Could you check a few things on this model? Use its own coordinates, in mm. A direction names the side the tool comes from. Coordinates: 2 decimals unless noted, no trailing zeros. Loops run counter-clockwise (first coordinate to the right, second up) from the corner with the lowest first, then second, coordinate; pieces in that order, holes last. Notation, with made-up numbers: (23.5, 75) - (44.5, 75) arc R23 cw to (44.5, 103) - close; hole circle Ø9 at (3, 29). An arc over 180 degrees is marked (long way). Use CSV: the item, a comma, the result in double quotes.
from build123d import *

# Parameters (mm, degrees)
SKETCH1_W               = 139
SKETCH1_H               = 160
BOSS_EXTRUDE1_DEPTH     = 5
SKETCH2_W               = 16
SKETCH2_H               = 16
CUT_EXTRUDE1_DEPTH      = 107.090763029
SKETCH3_R               = 2.2
CUT_EXTRUDE2_DEPTH      = 107.090763029
SKETCH4_R               = 2.2
CUT_EXTRUDE3_DEPTH      = 107.090763029
LPATTERN1_COUNT         = 4
LPATTERN1_PITCH         = 35
MIRROR2_COPY_1_SKETCH_R = 2.2
MIRROR2_COPY_1_DEPTH    = 107.090763029
MIRROR2_COPY_2_SKETCH_R = 2.2
MIRROR2_COPY_2_DEPTH    = 107.090763029
MIRROR2_COPY_3_SKETCH_R = 2.2
MIRROR2_COPY_3_DEPTH    = 107.090763029
SKETCH5_R               = 2.2
CUT_EXTRUDE4_DEPTH      = 107.090763029
SKETCH10_W              = 109
SKETCH10_H              = 15
BOSS_EXTRUDE2_DEPTH     = 5
SKETCH9_W               = 55
SKETCH9_H               = 104
CUT_EXTRUDE5_DEPTH      = 118.814472795
SKETCH11_W              = 55
SKETCH11_H              = 5
BOSS_EXTRUDE3_DEPTH     = 60
SKETCH12_R              = 1.375
CUT_EXTRUDE6_DEPTH      = 153.368796018
CUT_EXTRUDE7_REACH      = 154.369
SKETCH13_R              = 1.375
CUT_EXTRUDE8_REACH      = 196.821
SKETCH14_R              = 1.375
FILLET1_R               = 10
FILLET2_R               = 10


with BuildPart() as part:
    # Sketch1 → Boss-Extrude1 (new body)
    with BuildSketch(Plane(origin=(0, 0, 0), x_dir=(1, 0, 0), z_dir=(0, 1, 0))):
        Rectangle(SKETCH1_W, SKETCH1_H)
    extrude(amount=BOSS_EXTRUDE1_DEPTH)

    # Sketch2 → Cut-Extrude1 (cut, through all)
    with BuildSketch(Plane(origin=(0, 5, 0), x_dir=(1, 0, 0), z_dir=(0, 1, 0))):
        with Locations((-61.5, -72)):
            Rectangle(SKETCH2_W, SKETCH2_H)
    cut_extrude1 = extrude(amount=-CUT_EXTRUDE1_DEPTH, mode=Mode.SUBTRACT)

    # Mirror1: Cut-Extrude1 across plane
    add(cut_extrude1.mirror(Plane(origin=(0, 0, 0), x_dir=(0, 0, 1), z_dir=(1, 0, 0))), mode=Mode.SUBTRACT)

    # Sketch3 → Cut-Extrude2 (cut, through all)
    with BuildSketch(Plane(origin=(0, 5, 0), x_dir=(1, 0, 0), z_dir=(0, 1, 0))):
        with Locations(Location((0, -72.5, 0), (0, 0, 270))):
            Circle(SKETCH3_R)
        with Locations(Location((-25, -72.5, 0), (0, 0, 270))):
            Circle(SKETCH3_R)
        with Locations(Location((25, -72.5, 0), (0, 0, 270))):
            Circle(SKETCH3_R)
    extrude(amount=-CUT_EXTRUDE2_DEPTH, mode=Mode.SUBTRACT)

    # Sketch4 → Cut-Extrude3 (cut, through all)
    with BuildSketch(Plane(origin=(0, 5, 0), x_dir=(1, 0, 0), z_dir=(0, 1, 0))):
        with Locations(Location((-62, -49, 0), (0, 0, 270))):
            Circle(SKETCH4_R)
    cut_extrude3 = extrude(amount=-CUT_EXTRUDE3_DEPTH, mode=Mode.SUBTRACT)

    # LPattern1: Cut-Extrude3 ×4
    with Locations(*[(0, 0, -i * LPATTERN1_PITCH) for i in range(1, LPATTERN1_COUNT)]):
        add(cut_extrude3, mode=Mode.SUBTRACT)

    # Mirror2: Cut-Extrude3 across plane
    add(cut_extrude3.mirror(Plane(origin=(0, 0, 0), x_dir=(0, 0, 1), z_dir=(1, 0, 0))), mode=Mode.SUBTRACT)

    # Mirror2 copy 1 sketch → Mirror2 copy 1 (cut, through all)
    with BuildSketch(Plane(origin=(0, 5, -35), x_dir=(-1, 0, 0), z_dir=(0, 1, 0))):
        with Locations((-62, 49)):
            Circle(MIRROR2_COPY_1_SKETCH_R)
    extrude(amount=-MIRROR2_COPY_1_DEPTH, mode=Mode.SUBTRACT)

    # Mirror2 copy 2 sketch → Mirror2 copy 2 (cut, through all)
    with BuildSketch(Plane(origin=(0, 5, -70), x_dir=(-1, 0, 0), z_dir=(0, 1, 0))):
        with Locations((-62, 49)):
            Circle(MIRROR2_COPY_2_SKETCH_R)
    extrude(amount=-MIRROR2_COPY_2_DEPTH, mode=Mode.SUBTRACT)

    # Mirror2 copy 3 sketch → Mirror2 copy 3 (cut, through all)
    with BuildSketch(Plane(origin=(0, 5, -105), x_dir=(-1, 0, 0), z_dir=(0, 1, 0))):
        with Locations((-62, 49)):
            Circle(MIRROR2_COPY_3_SKETCH_R)
    extrude(amount=-MIRROR2_COPY_3_DEPTH, mode=Mode.SUBTRACT)

    # Sketch5 → Cut-Extrude4 (cut, through all)
    with BuildSketch(Plane(origin=(0, 5, 0), x_dir=(1, 0, 0), z_dir=(0, 1, 0))):
        with Locations(Location((-47.5, -32, 0), (0, 0, 270))):
            Circle(SKETCH5_R)
        with Locations(Location((-47.5, -7, 0), (0, 0, 270))):
            Circle(SKETCH5_R)
    cut_extrude4 = extrude(amount=-CUT_EXTRUDE4_DEPTH, mode=Mode.SUBTRACT)

    # Mirror3: Cut-Extrude4 across plane
    add(cut_extrude4.mirror(Plane(origin=(0, 0, 0), x_dir=(0, 0, 1), z_dir=(1, 0, 0))), mode=Mode.SUBTRACT)

    # Sketch10 → Boss-Extrude2 (add)
    with BuildSketch(Plane(origin=(0, 5, 0), x_dir=(1, 0, 0), z_dir=(0, 1, 0))):
        with Locations((0, 87.5)):
            Rectangle(SKETCH10_W, SKETCH10_H)
    extrude(amount=-BOSS_EXTRUDE2_DEPTH)

    # Sketch9 → Cut-Extrude5 (cut, through all)
    with BuildSketch(Plane(origin=(0, 5, 0), x_dir=(1, 0, 0), z_dir=(0, 1, 0))):
        with Locations((0, 33)):
            Rectangle(SKETCH9_W, SKETCH9_H)
    extrude(amount=-CUT_EXTRUDE5_DEPTH, mode=Mode.SUBTRACT)

    # Sketch11 → Boss-Extrude3 (add)
    with BuildSketch(Plane(origin=(0, 5, 0), x_dir=(1, 0, 0), z_dir=(0, 1, 0))):
        with Locations((0, 87.5)):
            Rectangle(SKETCH11_W, SKETCH11_H)
        with Locations((0, -21.5)):
            Rectangle(SKETCH11_W, SKETCH11_H)
    extrude(amount=BOSS_EXTRUDE3_DEPTH)

    # Sketch12 → Cut-Extrude6 (cut, through all)
    with BuildSketch(Plane.XY.offset(24)):
        with Locations((-22.5, 35)):
            Circle(SKETCH12_R)
        with Locations((22.5, 35)):
            Circle(SKETCH12_R)
    extrude(amount=-CUT_EXTRUDE6_DEPTH, mode=Mode.SUBTRACT)

    # Sketch13 → Cut-Extrude7 (cut, up to next)
    with BuildSketch(Plane.XY.offset(24), mode=Mode.PRIVATE) as cut_extrude7_sk1:
        with Locations((-22.5, 57)):
            Circle(SKETCH13_R)
    cut_extrude7_tool1 = extrude(cut_extrude7_sk1.sketch, amount=-CUT_EXTRUDE7_REACH, mode=Mode.PRIVATE) & part.part
    # Sketch13 → Cut-Extrude7 (cut, up to next)
    with BuildSketch(Plane.XY.offset(24), mode=Mode.PRIVATE) as cut_extrude7_sk2:
        with Locations((22.5, 57)):
            Circle(SKETCH13_R)
    cut_extrude7_tool2 = extrude(cut_extrude7_sk2.sketch, amount=-CUT_EXTRUDE7_REACH, mode=Mode.PRIVATE) & part.part
    add(cut_extrude7_tool1.solids().sort_by_distance((-22.5, 57, 24))[0], mode=Mode.SUBTRACT)
    add(cut_extrude7_tool2.solids().sort_by_distance((22.5, 57, 24))[0], mode=Mode.SUBTRACT)

    # Sketch14 → Cut-Extrude8 (cut, up to next)
    with BuildSketch(Plane(origin=(0, 0, -90), x_dir=(-1, 0, 0), z_dir=(0, 0, -1)), mode=Mode.PRIVATE) as cut_extrude8_sk1:
        with Locations((-22.5, 53.5)):
            Circle(SKETCH14_R)
    cut_extrude8_tool1 = extrude(cut_extrude8_sk1.sketch, amount=-CUT_EXTRUDE8_REACH, mode=Mode.PRIVATE) & part.part
    # Sketch14 → Cut-Extrude8 (cut, up to next)
    with BuildSketch(Plane(origin=(0, 0, -90), x_dir=(-1, 0, 0), z_dir=(0, 0, -1)), mode=Mode.PRIVATE) as cut_extrude8_sk2:
        with Locations((22.5, 53.5)):
            Circle(SKETCH14_R)
    cut_extrude8_tool2 = extrude(cut_extrude8_sk2.sketch, amount=-CUT_EXTRUDE8_REACH, mode=Mode.PRIVATE) & part.part
    add(cut_extrude8_tool1.solids().sort_by_distance((22.5, 53.5, -90))[0], mode=Mode.SUBTRACT)
    add(cut_extrude8_tool2.solids().sort_by_distance((-22.5, 53.5, -90))[0], mode=Mode.SUBTRACT)

    # Fillet1
    fillet1_edges = [part.edges().sort_by_distance(p)[0] for p in [
        (0, 5, 24),
    ]]
    fillet(fillet1_edges, radius=FILLET1_R)

    # Fillet2
    # the kernel refuses this fillet: 10 mm, written as the material it adds along each edge
    with BuildSketch(Plane(origin=(27.5, 5, -90), x_dir=(0, 0, -1), z_dir=(-1, 0, 0))) as fillet2_piece_1:
        with BuildLine():
            CenterArc((10, -8.660254038), FILLET2_R, 120, 60)
            Line((0, -8.660254038), (-0.2, -8.660254038))
            Line((-0.2, -8.660254038), (-0.2, 0))
            Line((-0.2, 0), (0, 0.2))
            ThreePointArc((0, 0.2), (2.5, 0.2), (4.9, 0.173205081))
            Line((4.9, 0.173205081), (5, 0))
        make_face()
    extrude(amount=55)


solid = part.part
(1) Suppose I cut it at D-D (z = -31). Write out the boundary of the cut face in (x, y), plus the area to 3 significant figures.
Computed:
outline,"(-69.5, 0) - (-27.5, 0) - (-27.5, 5) - (-69.5, 5) - close; (27.5, 0) - (69.5, 0) - (69.5, 5) - (27.5, 5) - close"
area,"420 mm²"
(2) Suppose I cut it at A-A (z = -56). Write out the boundary of the cut face in (x, y), plus the area to 3 significant figures.
Computed:
outline,"(-69.5, 0) - (-64.2, 0) - (-64.2, 5) - (-69.5, 5) - close; (-59.8, 0) - (-27.5, 0) - (-27.5, 5) - (-59.8, 5) - close; (27.5, 0) - (59.8, 0) - (59.8, 5) - (27.5, 5) - close; (64.2, 0) - (69.5, 0) - (69.5, 5) - (64.2, 5) - close"
area,"376 mm²"
(3) Suppose I cut it at B-B (x = 47.5). Write out the boundary of the cut face in (y, z).
Computed:
outline,"(0, -95) - (5, -95) - (5, 4.8) - (0, 4.8) - close; (0, 9.2) - (5, 9.2) - (5, 29.8) - (0, 29.8) - close; (0, 34.2) - (5, 34.2) - (5, 80) - (0, 80) - close"
(4) Which directions (+Z, -Z, +X, -X, +Y, -Y) give clear straight access to the entire face, cutting with the end or side of a thin tool? Please do faces 1 (the face through (53.5, 3, 72)), 2 (the face through (0, 40, 24)), 3 (the face through (-27.5, 35, -88)), 4 (the face through (27.5, 3, -32)).
Computed:
face 1,"+Z, +X, +Y, -Y"
face 2,"+Z, +X, -X, +Y"
face 3,"+Z, -Z, -X, +Y"
face 4,"+Y, -Y"
(5) Suppose I cut it at C-C (y = 18.5). Write out the boundary of the cut face in (x, z), plus the area to 3 significant figures.
Computed:
outline,"(-27.5, -90) - (27.5, -90) - (27.5, -85) - (-27.5, -85) - close; (-27.5, 19) - (27.5, 19) - (27.5, 24) - (-27.5, 24) - close"
area,"550 mm²"
(6) Will these pins go through, and if not, where does the flat tip stop? pin 1 (4 mm diameter, centred on y = 1.5, z = 72.5, fed in from +X); pin 2 (7 mm diameter, centred on x = -62, z = -21, fed in from +Y); pin 3 (4 mm diameter, centred on x = 62.5, y = 3.5, fed in from -Z).
Computed:
pin 1,"stops at x = 53.5"
pin 2,"stops at y = 5"
pin 3,"stops at z = -80"
(7) Please list where these lines run through material, in increasing order: line 1 (Z direction, x = 62, y = 3); line 2 (X direction, y = 2.2, z = 32); line 3 (Z direction, x = -6, y = 41).
Computed:
line 1,"z = -80 to -58.2, -53.8 to -23.2, -18.8 to 11.8, 16.2 to 46.8, 51.2 to 64"
line 2,"x = -69.5 to -49.7, -45.3 to 45.3, 49.7 to 69.5"
line 3,"z = -90 to -85, 19 to 24"
(8) Thinking about a two-plate mould opening in X: for faces 5 (the face through (0.39, 7.85, 27.01)), 6 (the face through (54.5, 3, -87)), 7 (the face through (60.98, 2.54, -57.95)), which applies, +X half, -X half, draft (parallel to the pull), parting line (faces both ways), or undercut?
Computed:
face 5,"draft"
face 6,"+X half"
face 7,"undercut"
